Source: CAD feature listing. Evaluate the final solid. Frame: model axes, mm. A direction names the side the tool comes from. Coordinates: 2 decimals unless noted, no trailing zeros. Loops run counter-clockwise (first coordinate to the right, second up) from the corner with the lowest first, then second, coordinate; pieces in that order, holes last. Notation, with made-up numbers: M -33.5,-14.75 L 14.5,-14.75 A17 ccw 14.5,-0.75 Z; hole C 74,7.25 d8. An arc over 180 degrees is marked long. One line per question, with ' | ' between items. Start each with the question number.
1. Mould query, pull axis X, two halves, no side actions, for faces 1 (the flat face through (-1, -6, 19.304)), 2 (the flat face through (3.131, -5.525, 10.161)), 3 (the cylindrical face through (1.4, 2.19, 24.31)), 4 (the flat face through (-3.131, 5.525, 10.161)). Classes: pulls with the +X half, pulls with the -X half, needs draft (parallel to the pull), parting line crosses it, or undercut.
2. Section query A-A, the plane y = 0. Output: boundary loops of the cut face in (x, z) (3 decimals), and give its area (3 significant figures).
3. Ray query, probe 1 along Y at (x, z) = (0, 23.35); probe 2 along X at (y, z) = (0, 11.5) (3 decimals); probe 3 along Z at (x, y) = (-4.5, 4). Return the intervals inside material, ascending.
4. Pin query (flat end, axial travel): P1, Ø3.5, axis at y = -0.5, z = 10, coming from the -X side; P2, Ø2, axis at y = -1, z = 13.5, coming from the +X side; P3, Ø5, axis at x = -3.5, y = -5.5, coming from the +Z side. Return the tip coordinate at first contact, or that it passes through.
5. Access query for faces 5 (the flat face through (6.35, 0, 10)), 6 (the cylindrical face through (-1.266, -5.703, 19.93)), 7 (the flat face through (-6.35, 0, 10)). Directions: +Z, -Z, +X, -X, +Y, -Y. A direction counts if a zero-diameter tool reaches every point of the face in a straight line with its end or side. Return the directions, or none.
6. Section query C-C, the plane x = -4. Output: boundary loops of the cut face in (y, z), and give its area (3 significant figures).
7. Section query B-B, the plane z = 14. Output: boundary loops of the cut face in (x, y) (3 decimals), and give its area (3 significant figures).
8. Section query D-D, the plane y = -1.75. State how many separate pieces and enclosed holes the cut face has, and give its area (3 significant figures).
```python
from build123d import *

# Parameters (mm, degrees)
BOSS_EXTRU_1_DEPTH      = 19.304
ESQUISSE2_R             = 7.62
BOSS_EXTRU_2_DEPTH      = 1.27
ESQUISSE3_R             = 5.842
BOSS_EXTRU_3_DEPTH      = 1.27
ESQUISSE4_R             = 6.35
BOSS_EXTRU_4_DEPTH      = 1.27
ESQUISSE5_R             = 2.525
ENL_V_MAT_EXTRU_1_DEPTH = 25.357527297
ESQUISSE7_R             = 2.95
ESQUISSE7_R_2           = 2.6
BOSS_EXTRU_6_DEPTH      = 5
ESQUISSE8_R             = 1.55
ENL_V_MAT_EXTRU_2_DEPTH = 5


with BuildPart() as part:
    # Esquisse1 → Boss.-Extru.1 (new body)
    with BuildSketch(Plane.XY):
        Polygon((0, 7.332348419), (-6.35, 3.666174209), (-6.35, -3.666174209), (0, -7.332348419), (6.35, -3.666174209), (6.35, 3.666174209), align=None)
    extrude(amount=BOSS_EXTRU_1_DEPTH)

    # Esquisse2 → Boss.-Extru.2 (add)
    with BuildSketch(Plane.XY):
        Circle(ESQUISSE2_R)
    extrude(amount=BOSS_EXTRU_2_DEPTH)

    # Esquisse3 → Boss.-Extru.3 (add)
    with BuildSketch(Plane.XY.offset(19.304)):
        Circle(ESQUISSE3_R)
    extrude(amount=BOSS_EXTRU_3_DEPTH)

    # Esquisse4 → Boss.-Extru.4 (add)
    with BuildSketch(Plane.XY.offset(20.574)):
        with Locations(Location((0, 0, 0), (0, 0, 180))):
            Circle(ESQUISSE4_R)
    extrude(amount=BOSS_EXTRU_4_DEPTH)

    # Esquisse5 → Enlèv. mat.-Extru.1 (cut, through all)
    with BuildSketch(Plane.XY):
        Circle(ESQUISSE5_R)
    extrude(amount=ENL_V_MAT_EXTRU_1_DEPTH, mode=Mode.SUBTRACT)

    # Esquisse7 → Boss.-Extru.6 (add)
    with BuildSketch(Plane.XY.offset(21.844)):
        Circle(ESQUISSE7_R)
        Circle(ESQUISSE7_R_2, mode=Mode.SUBTRACT)
    extrude(amount=BOSS_EXTRU_6_DEPTH)

    # Esquisse8 → Enlèv. mat.-Extru.2 (cut)
    with BuildSketch(Plane(origin=(-3.175, -5.499261314, 0), x_dir=(0.8660254037844417, -0.49999999999999495, 0), z_dir=(-0.49999999999999495, -0.8660254037844417, 0))):
        with Locations((0, 24.384)):
            Circle(ESQUISSE8_R)
    extrude(amount=-ENL_V_MAT_EXTRU_2_DEPTH, mode=Mode.SUBTRACT)


solid = part.part
```
Taken from the geometry:
1) face 1: needs draft | face 2: pulls with the +X half | face 3: undercut | face 4: pulls with the -X half
2) outline: M -7.62,0 L -2.525,0 L -2.525,21.844 L -2.6,21.844 L -2.6,26.844 L -2.95,26.844 L -2.95,21.844 L -6.35,21.844 L -6.35,20.574 L -5.842,20.574 L -5.842,19.304 L -6.35,19.304 L -6.35,1.27 L -7.62,1.27 Z; M 2.525,0 L 7.62,0 L 7.62,1.27 L 6.35,1.27 L 6.35,19.304 L 5.842,19.304 L 5.842,20.574 L 6.35,20.574 L 6.35,21.844 L 2.95,21.844 L 2.95,26.844 L 2.6,26.844 L 2.6,21.844 L 2.525,21.844 Z | area: 173 mm^2
3) probe 1: -2.95 to -2.6, 2.6 to 2.95 | probe 2: -6.35 to -2.525, 2.525 to 6.35 | probe 3: 0 to 19.3, 20.57 to 21.84
4) P1: x = -6.35 | P2: x = 6.35 | P3: z = 21.84
5) face 5: +Z, +X, +Y, -Y | face 6: none | face 7: +Z, -X, +Y, -Y
6) outline: M -6.49,0 L 6.49,0 L 6.49,1.27 L 5.02,1.27 L 5.02,19.3 L 4.26,19.3 L 4.26,20.57 L 4.93,20.57 L 4.93,21.84 L -4.93,21.84 L -4.93,20.57 L -4.26,20.57 L -4.26,19.3 L -5.02,19.3 L -5.02,1.27 L -6.49,1.27 Z | area: 221 mm^2
7) outline: M -6.35,-3.666 L 0,-7.332 L 6.35,-3.666 L 6.35,3.666 L 0,7.332 L -6.35,3.666 Z; hole C 0,0 d5.05 | area: 120 mm^2
8) separate pieces: 3 | enclosed holes: 0 | area: 201 mm^2
